Input: dimensioned drawing with shaded views. Units: mm. Origin: part minimum x, y, z. A direction names the side the tool comes from. Round coordinates to 2 decimals unless told otherwise and drop trailing zeros. Write each loop counter-clockwise with the first axis right and the second up, starting at its lowest first coordinate (ties: lowest second). Pieces come first, ordered by that corner, then holes. Notation, with made-up numbers: M -19.5,-19.75 L -12.5,-19.75 A13 cw -12.5,4.25 Z; hole C -39.5,84 d6. An arc over 180 degrees is marked long. Answer in a Markdown table with one row per item. Add a question column.
Item 1: Contact query for a flat-ended pin moving along its axis: pin 1 (8 mm diameter, centred on x = 51.5, z = 9, fed in from -Y). Output: stop coordinate, or through.
Item 2: Set-up query: the marked faces 5 and 6. Return all of +Z, -Z, +X, -X, +Y, -Y with unobstructed straight access to the full face (end or side cutting, diameter ignored); none if empty.
Item 3: Cut plane A-A on z = 54.5. Return loops of the section in (x, y), and give its area (3 significant figures).
Item 4: Material intervals for probe 1 along X at (y, z) = (36.5, 19.5); probe 2 along Y at (x, z) = (51.5, 35); probe 3 along X at (y, z) = (22.5, 5), sorted ascending.
Item 5: Cut plane B-B on x = 54. Return loops of the section in (y, z).
Item 6: Mould query, pull axis X, two halves, no side actions, for the marked faces 1, 2, 3 and 4. Classes: released by +X, released by -X, zero draft, split by the parting line, or undercut.
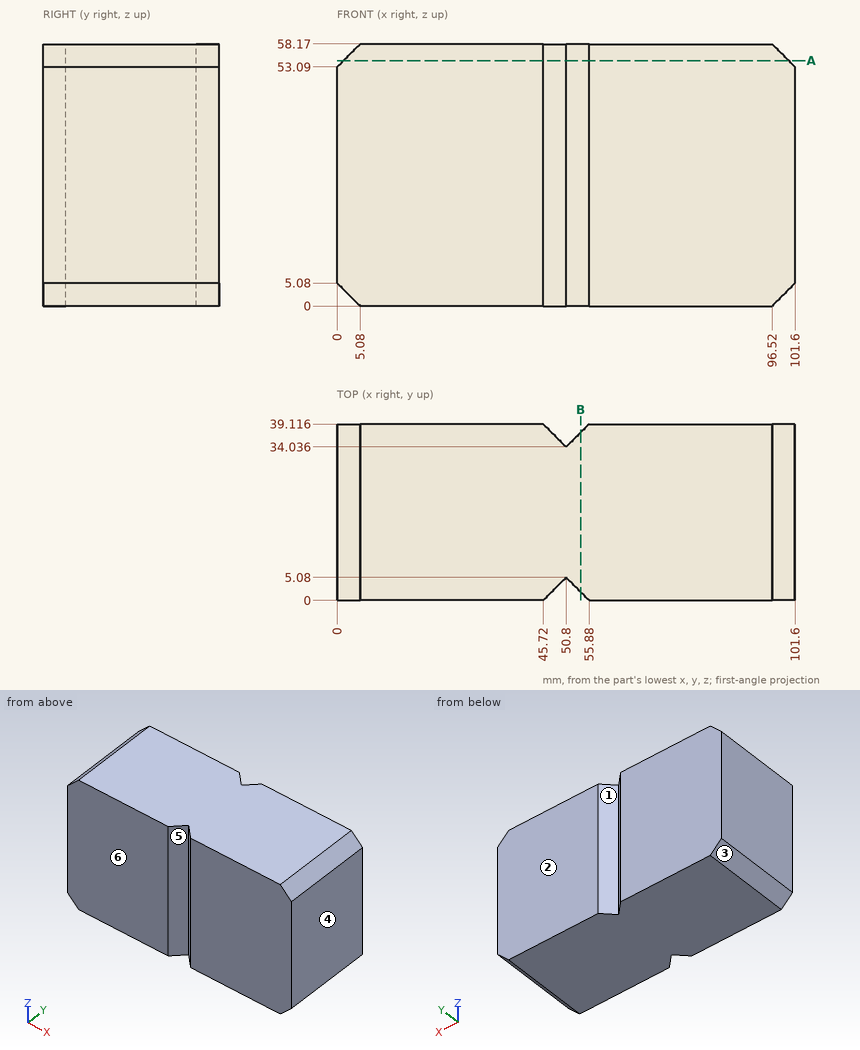
Results below:
| question | item | result |
|---|---|---|
| 1 | pin 1 | y = 0.38 |
| 2 | face 5 | +Z, -Z, -Y |
| 2 | face 6 | +Z, -Z, +X, -X, -Y |
| 3 | outline | M 1.41,0 L 45.72,0 L 50.8,5.08 L 55.88,0 L 100.19,0 L 100.19,39.12 L 55.88,39.12 L 50.8,34.04 L 45.72,39.12 L 1.41,39.12 Z |
| 3 | area | 3,810 mm2 |
| 4 | probe 1 | 0 to 48.34, 53.26 to 101.6 |
| 4 | probe 2 | 4.38 to 34.74 |
| 4 | probe 3 | 0.08 to 101.52 |
| 5 | outline | M 1.88,0 L 37.24,0 L 37.24,58.17 L 1.88,58.17 Z |
| 6 | face 1 | undercut |
| 6 | face 2 | zero draft |
| 6 | face 3 | released by -X |
| 6 | face 4 | released by +X |
